Verification items for the finished model (mm, model axes). Round coordinates to 2 decimals unless told otherwise and drop trailing zeros. Write each loop counter-clockwise with the first axis right and the second up, starting at its lowest first coordinate (ties: lowest second). Pieces come first, ordered by that corner, then holes. Notation, with made-up numbers: M 76.5,66.25 L 134.5,66.25 A10 ccw 134.5,71.25 Z; hole C 2.5,0 d2. An arc over 180 degrees is marked long. One line per question, with ' | ' between items. Start each with the question number.
Q1. Cross-section at A-A (z = 40). Record the boundary of the cut face in (x, y).
Q2. Cross-section at B-B (z = 31). Record the boundary of the cut face in (x, y).
Q3. Gauge pin test, flat ends, axial feed: pin 1 (1.5 mm diameter, centred on y = 3.5, z = 8.5, fed in from +X); pin 2 (2 mm diameter, centred on y = 3.5, z = 7.5, fed in from +X); pin 3 (2 mm diameter, centred on x = 0, y = 0, fed in from +Z). Record the tip position at first contact, or that the pin passes through.
Q4. Cross-section at C-C (x = -3.25). Record the boundary of the cut face in (y, z), then the cut area to 3 significant figures.
Q5. Thickness scan on line 1 along Y through (x, z) = (0, 7.25); line 2 along X through (y, z) = (1.25, 43); line 3 along X through (y, z) = (-4.25, 32). Record the ranges inside material, lowest first. Write a range as from..to.
from build123d import *

# Parameters (mm, degrees)
SKETCH_1_R             = 4.9
EXTRUDE_1_DEPTH        = 50
HOLE_WIZARD_M4_1_D     = 3.3
HOLE_WIZARD_M4_1_DEPTH = 11.5
HOLE_WIZARD_M4_1_TIP   = 0.991420021
HOLE_WIZARD_M4_2_D     = 3.3
HOLE_WIZARD_M4_2_DEPTH = 11.5
HOLE_WIZARD_M4_2_TIP   = 0.991420021


with BuildPart() as part:
    # 스케치1 → 보스-돌출1 (new body)
    with BuildSketch(Plane.XY):
        Circle(SKETCH_1_R)
    extrude(amount=EXTRUDE_1_DEPTH)

    # M4 나사 구멍1
    with Locations(Plane.XY.offset(50)):
        with Locations((0, 0)):
            Hole(HOLE_WIZARD_M4_1_D / 2, depth=HOLE_WIZARD_M4_1_DEPTH)
            with Locations((0, 0, -(HOLE_WIZARD_M4_1_DEPTH + HOLE_WIZARD_M4_1_TIP / 2))):  # 118° drill point
                Cone(0, HOLE_WIZARD_M4_1_D / 2, HOLE_WIZARD_M4_1_TIP, mode=Mode.SUBTRACT)

    # M4 나사 구멍2
    with Locations(Plane(origin=(0, 0, 0), x_dir=(-1, 0, 0), z_dir=(0, 0, -1))):
        with Locations((0, 0)):
            Hole(HOLE_WIZARD_M4_2_D / 2, depth=HOLE_WIZARD_M4_2_DEPTH)
            with Locations((0, 0, -(HOLE_WIZARD_M4_2_DEPTH + HOLE_WIZARD_M4_2_TIP / 2))):  # 118° drill point
                Cone(0, HOLE_WIZARD_M4_2_D / 2, HOLE_WIZARD_M4_2_TIP, mode=Mode.SUBTRACT)


solid = part.part
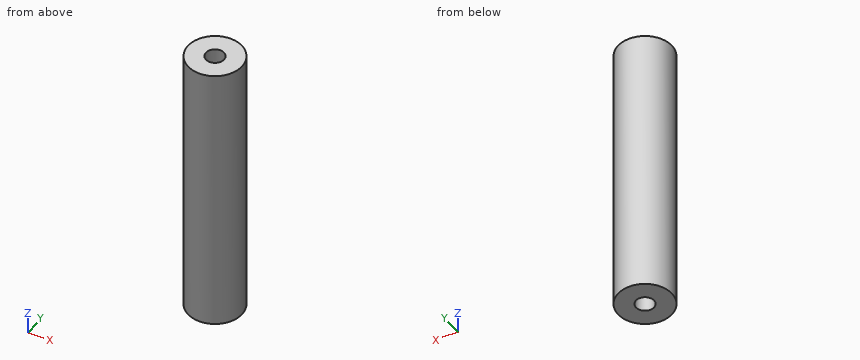
Determined:
1) outline: C 0,0 d9.8; hole C 0,0 d3.3
2) outline: C 0,0 d9.8
3) pin 1: stops at x = 4.06 | pin 2: stops at x = 4.21 | pin 3: stops at z = 38.11
4) outline: M -3.67,0 L 3.67,0 L 3.67,50 L -3.67,50 Z | area: 367 mm²
5) line 1: y = -4.9..-1.65, 1.65..4.9 | line 2: x = -4.74..-1.08, 1.08..4.74 | line 3: x = -2.44..2.44
